from build123d import *

# Parameters (mm, degrees)
F1_DEPTH = 40.03749


with BuildPart() as f1:
    # F0 (on Right) → F1 (new body)
    with BuildSketch(Plane.YZ):
        with BuildLine():
            ThreePointArc((44.5198227701, -1.7826942255), (44.5465801188, -0.8915256021), (44.5555004257, 0))
            ThreePointArc((44.5555004257, 0), (43.3760301156, 10.1839397872), (39.9000649082, 19.8287023908))
            Line((39.9000649082, 19.8287023908), (16.4275774694, 19.2902224238))
            ThreePointArc((16.4275774694, 19.2902224238), (25.6072357444, 2.2662942698), (44.5198227701, -1.7826942255))
        make_face()
        with BuildLine():
            ThreePointArc((39.9000649082, 19.8287023908), (43.3760301156, 10.1839397872), (44.5555004257, 0))
            ThreePointArc((44.5555004257, 0), (44.5465801188, -0.8915256021), (44.5198227701, -1.7826942255))
            ThreePointArc((44.5198227701, -1.7826942255), (57.4595301276, 6.3123736108), (62.5101083198, 20.7157693803))
            ThreePointArc((62.5101083198, 20.7157693803), (48.6974420854, 41.8425767898), (23.8043112787, 37.6636082011))
            ThreePointArc((23.8043112787, 37.6636082011), (33.0769232647, 29.8514616983), (39.9000649082, 19.8287023908))
        make_face()
        with BuildLine():
            Line((16.4275774694, 19.2902224238), (39.9000649082, 19.8287023908))
            ThreePointArc((39.9000649082, 19.8287023908), (33.0769232647, 29.8514616983), (23.8043112787, 37.6636082011))
            ThreePointArc((23.8043112787, 37.6636082011), (18.0440587641, 29.3087570216), (16.4275774694, 19.2902224238))
        make_face()
        with BuildLine():
            ThreePointArc((0, -44.5555004257), (30.8687850819, -32.1295926795), (44.5198227701, -1.7826942255))
            ThreePointArc((44.5198227701, -1.7826942255), (25.6072357444, 2.2662942698), (16.4275774694, 19.2902224238))
            Line((16.4275774694, 19.2902224238), (0, 18.9133590259))
            Line((0, 18.9133590259), (0, -44.5555004257))
        make_face()
        with BuildLine():
            ThreePointArc((16.4275774694, 19.2902224238), (18.0440587641, 29.3087570216), (23.8043112787, 37.6636082011))
            ThreePointArc((23.8043112787, 37.6636082011), (-2.5921293007, 44.4800346658), (-28.0181032693, 34.6435925876))
            ThreePointArc((-28.0181032693, 34.6435925876), (-22.0629919245, 27.4874750802), (-19.7900024173, 18.4593585764))
            Line((-19.7900024173, 18.4593585764), (0, 18.9133590259))
            Line((0, 18.9133590259), (16.4275774694, 19.2902224238))
        make_face()
        with BuildLine():
            ThreePointArc((-44.4751519011, -2.6745993272), (-30.5452492764, -32.4373298041), (0, -44.5555004257))
            Line((0, -44.5555004257), (0, 18.9133590259))
            Line((0, 18.9133590259), (-19.7900024173, 18.4593585764))
            ThreePointArc((-19.7900024173, 18.4593585764), (-19.7858629772, 18.2187543647), (-19.7844831034, 17.9781185038))
            ThreePointArc((-19.7844831034, 17.9781185038), (-27.304798405, 1.8833687428), (-44.4751519011, -2.6745993272))
        make_face()
        with BuildLine():
            ThreePointArc((-19.7900024173, 18.4593585764), (-22.0629919245, 27.4874750802), (-28.0181032693, 34.6435925876))
            ThreePointArc((-28.0181032693, 34.6435925876), (-35.3877865562, 27.0720738186), (-40.7673873733, 17.9781185038))
            Line((-40.7673873733, 17.9781185038), (-19.7900024173, 18.4593585764))
        make_face()
        with BuildLine():
            ThreePointArc((-40.7673873733, 17.9781185038), (-35.3877865562, 27.0720738186), (-28.0181032693, 34.6435925876))
            ThreePointArc((-28.0181032693, 34.6435925876), (-59.9663230472, 26.444708171), (-44.4751519011, -2.6745993272))
            ThreePointArc((-44.4751519011, -2.6745993272), (-43.8543762233, 7.8731381447), (-40.7673873733, 17.9781185038))
        make_face()
        with BuildLine():
            ThreePointArc((-40.7673873733, 17.9781185038), (-43.8543762233, 7.8731381447), (-44.4751519011, -2.6745993272))
            ThreePointArc((-44.4751519011, -2.6745993272), (-27.304798405, 1.8833687428), (-19.7844831034, 17.9781185038))
            ThreePointArc((-19.7844831034, 17.9781185038), (-19.7858629772, 18.2187543647), (-19.7900024173, 18.4593585764))
            Line((-19.7900024173, 18.4593585764), (-40.7673873733, 17.9781185038))
        make_face()
    extrude(amount=-F1_DEPTH)


solid = f1.part
For this review, take the finished solid that the model builds, in its own axes (mm). Round coordinates to 2 decimals unless told otherwise and drop trailing zeros. Order: outer loops, then holes, each group sorted by start corner. A loop starts at its lowest first (then second) coordinate and runs counter-clockwise, first axis right, second up. Notation, with made-up numbers: (-12, 26.25) -> (19, 26.25) arc R23 ccw to (19, 34.25) -> close; hole circle Ø4 at (82, 72.25). An arc over 180 degrees is marked (long way). Put each result on its own line as item: value.
Q1. Add section B-B on z = -21.5. Write out the cut boundary in (x, y), plus the area to 3 significant figures.
Check result:
outline: (-40.04, -39.02) -> (0, -39.02) -> (0, 39.02) -> (-40.04, 39.02) -> close
area: 3,120 mm2
Q2. Insertion check: pin 1 Ø4 at (x, y) = (-11.5, -24) entering from +Z; pin 2 Ø12 at (x, y) = (-24.5, 34.5) entering from -Z; pin 3 Ø1.5 at (x, y) = (-25.5, 10.5) entering from +Z. Each pin has a flat end and moves straight along its axis. Give the tip position at first contact, or say it passes through.
Check result:
pin 1: z = 38.75
pin 2: z = -34.25
pin 3: z = 43.48
Q3. For probe 1 along Z at (x, y) = (-20, 0.5); probe 2 along Y at (x, z) = (-8.5, 35.5); probe 3 along Y at (x, z) = (-4.5, 36), list the stretches that pass through material, from the lowest coordinate up. Write a range as [from, to].
Check result:
probe 1: [-44.55, 44.55]
probe 2: [-52.31, -29.22], [-26.92, 57.15]
probe 3: [-51.51, -30.02], [-26.25, 56.72]
Q4. Mouldability with a two-part tool opening along Y and no side actions: class faces 1 (the cylindrical face through (-19.738, -59.746, 26.928)), 2 (the flat face through (-40.037, 0, 1)), 3 (the cylindrical face through (-19.7, -2.2, 44.5)) as pulls with the +Y half, pulls with the -Y half, needs draft (parallel to the pull), parting line crosses it, or undercut.
Check result:
face 1: undercut
face 2: needs draft
face 3: undercut
Q5. Add section A-A on x = -15. Write out the cut boundary in (y, z), plus the area to 3 significant figures.
Check result:
outline: (-44.48, -2.67) arc R44.56 ccw to (44.52, -1.78) arc R23.06 ccw (long way) to (23.8, 37.66) arc R44.56 ccw to (-28.02, 34.64) arc R20.98 ccw (long way) to start
area: 7,930 mm2
Q6. Add section C-C on y = -8. Write out the cut boundary in (x, z).
Check result:
outline: (-40.04, -43.83) -> (0, -43.83) -> (0, 43.83) -> (-40.04, 43.83) -> close
